Verification items for the finished model (mm, model axes). Coordinates: 2 decimals unless noted, no trailing zeros. Loops run counter-clockwise (first coordinate to the right, second up) from the corner with the lowest first, then second, coordinate; pieces in that order, holes last. Notation, with made-up numbers: (-30.5, 7) - (24.5, 7) arc R24 ccw to (24.5, 24) - close; hole circle Ø10 at (52.5, -26). An arc over 180 degrees is marked (long way). Answer as CSV lines item,"result". Start each with the question number.
1. Cross-section at B-B (x = -7). Enter the section's corners in (y, z), plus the area to 3 significant figures.
2. Gauge pin test, flat ends, axial feed: P1, Ø2, axis at x = 24.5, z = 1, coming from the -Y side; P2, Ø1, axis at y = -12, z = 2.5, coming from the -X side. Record the tip position at first contact, or that the pin passes through.
3. Cross-section at A-A (z = 2.95). Enter the section's corners in (x, y) (1 decimal), plus the area to 3 significant figures.
4. Cross-section at C-C (y = 27). Enter the section's corners in (x, z), plus the area to 3 significant figures.
5. Material ranges on line 1 (Y direction, x = 0, z = 2.5); line 2 (Y direction, x = -2, z = 0.4); line 3 (X direction, y = -16.5, z = 3.5), recorded low to high. Write a range as [from, to].
```python
from build123d import *

# Parameters (mm, degrees)
F1_DEPTH = 4.7625


with BuildPart() as f1:
    # F0 (on Top) → F1 (new body)
    with BuildSketch(Plane.XY):
        with BuildLine():
            ThreePointArc((-18.7669216404, 33.1573921192), (-19.1910172412, -32.9137487572), (38.1, 0))
            ThreePointArc((38.1, 0), (26.8100597322, 27.0708458891), (-0.3688030002, 38.0982149759))
            Line((-0.3688030002, 38.0982149759), (-0.046100375, 4.762276872))
            ThreePointArc((-0.046100375, 4.762276872), (3.3512574665, 3.3838557361), (4.7625, 0))
            ThreePointArc((4.7625, 0), (-2.3988771551, -4.1142185946), (-2.345865205, 4.1446740149))
            Line((-2.345865205, 4.1446740149), (-18.7669216404, 33.1573921192))
        make_face()
        with BuildLine():
            Line((-18.7669216404, 33.1573921192), (-0.3688030002, 38.0982149759))
            ThreePointArc((-0.3688030002, 38.0982149759), (-9.8816457134, 36.7962372804), (-18.7669216404, 33.1573921192))
        make_face()
        with BuildLine():
            Line((-0.046100375, 4.762276872), (-0.3688030002, 38.0982149759))
            Line((-0.3688030002, 38.0982149759), (-18.7669216404, 33.1573921192))
            Line((-18.7669216404, 33.1573921192), (-2.345865205, 4.1446740149))
            ThreePointArc((-2.345865205, 4.1446740149), (-1.2352057142, 4.59952966), (-0.046100375, 4.762276872))
        make_face()
    extrude(amount=F1_DEPTH)


solid = f1.part
```
Values follow:
1,outline,"(-37.45, 0) - (37.45, 0) - (37.45, 4.76) - (-37.45, 4.76) - close"
1,area,"357 mm²"
2,P1,"stops at y = -29.99"
2,P2,"stops at x = -36.32"
3,outline,"circle Ø76.2 at (0, 0); hole circle Ø9.5 at (0, 0)"
3,area,"4,490 mm²"
4,outline,"(-26.88, 0) - (26.88, 0) - (26.88, 4.76) - (-26.88, 4.76) - close"
4,area,"256 mm²"
5,line 1,"y = [-38.1, -4.76], [4.76, 38.1]"
5,line 2,"y = [-38.05, -4.32], [4.32, 38.05]"
5,line 3,"x = [-34.34, 34.34]"
